Solid Edge part; units mm, degrees
sketch "Sketch1" plane through (0, 0, 0) normal (0, 0, 1) x (1, 0, 0)
  circle A0 centre (0, 0) radius 101.5
extrude "Protrusion1" add sketch "Sketch1" against normal blind 19
sketch "Sketch2" plane through (0, 0, 0) normal (0, 0, 1) x (1, 0, 0)
  circle A0 centre (0, 0) radius 32
extrude "ExtrudedProtrusion_2" add sketch "Sketch2" along normal blind 51
sketch "Sketch3" plane through (0, 0, 0) normal (0, 0, 1) x (1, 0, 0)
  circle A0 centre (0, 0) radius 16
extrude "ExtrudedCutout_1" cut sketch "Sketch3" along normal blind 51 and the other way blind 19
sketch "Sketch4" plane through (0, 0, 0) normal (0, 0, 1) x (1, 0, 0)
  circle A0 centre (0, 86) radius 8
extrude "ExtrudedCutout_2" cut sketch "Sketch4" against normal blind 19
pattern_circular "Pattern1" count 6 over 360 about axis through (0, 0, 0) along (0, 0, -1) of "ExtrudedCutout_2"
sketch "Sketch5" plane through (0, 0, 0) normal (-0.866, -0.5, 0) x (0, 0, -1)
  line L0 (-17.8752, -123.9402) -> (-51, -32)
  line L1 (-51, -32) -> (-51, -21.8003)
  line L2 (19, -21.8003) -> (-51, -21.8003)
  line L3 (19, -117.5) -> (19, -21.8003)
  arc A0 (19, -117.5) -> (-17.8752, -123.9402) centre (0, -117.5) cw
extrude "Protrusion_3" add sketch "Sketch5" along normal mid plane 16
sketch "Sketch6" plane through (0, 0, 0) normal (-0.866, -0.5, 0) x (0, 0, -1)
  circle A0 centre (0, -117.5) radius 6.5
extrude "Cutout_3" cut sketch "Sketch6" along normal mid plane 16
pattern_circular "Pattern2" count 3 over 360 about axis through (0, 0, 0) along (0, 0, -1) of "Protrusion_3", "Cutout_3"
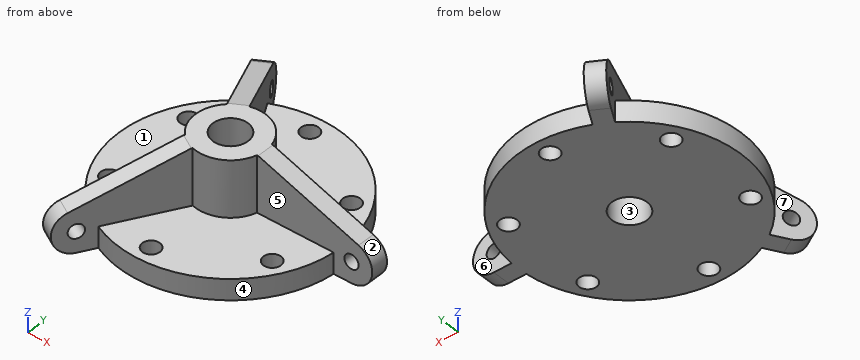
Design review of the part built by this model. Coordinates are the model's own, in mm. Face numbers are marked on the shaded views. A direction names the side the tool comes from. Round coordinates to 2 decimals unless told otherwise and drop trailing zeros. Write each loop counter-clockwise with the first axis right and the second up, starting at its lowest first coordinate (ties: lowest second). Pieces come first, ordered by that corner, then holes. Notation, with made-up numbers: M -30.75,-34 L -8.75,-34 A13 ccw -8.75,-30 Z; hole C -4,-28 d5. An arc over 180 degrees is marked long. One line per item, written item: value. Start each with the question number.
1. Take a section at A-A on y = 0. State the section outline as (x, z) points.
2. Take a section at C-C on z = 13. State the section outline as (x, y) points, then the cut area to 3 significant figures.
3. To check wall thickness, follow probe 1 along Y at (x, z) = (0, -14); probe 2 along X at (y, z) = (-46.5, -4); probe 3 along Z at (x, y) = (92.5, 38.5). State the ranges of each line that lie inside material, in increasing order. Write a range as from..to.
4. Draft analysis for pull direction X (two halves, no side actions). For the marked faces 1, 2, 3 and 4, state which applies: pulls with the +X half, pulls with the -X half, needs draft (parallel to the pull), parting line crosses it, or undercut.
5. Take a section at D-D on y = 43. State the section outline as (x, z) points.
6. Clearance check with flat-ended pins moving along their axes: P1, Ø12, axis at x = 54.5, z = 17, coming from the -Y side; P2, Ø9.5, axis at x = 0, y = -86, coming from the +Z side; P3, Ø8, axis at x = 47.5, z = -9, coming from the +Y side; P4, Ø21, axis at x = 74.48, y = -43, coming from the -Z side. State where each tip first meets the part, or that it passes through.
7. Take a section at B-B on x = 0. State the section outline as (y, z) points, then the cut area to 3 significant figures.
8. For the marked faces 5, 6 and 7, list the 3-axis set-ups (+Z, -Z, +X, -X, +Y, -Y) from which the entire face can be reached by the end or side of a thin tool; tool diameter is ignored.
Computed:
1. outline: M -101.5,-19 L -16,-19 L -16,51 L -32,51 L -32,0 L -101.5,0 Z; M 16,-19 L 117.5,-19 A19 ccw 123.94,17.88 L 32,51 L 16,51 Z; hole C 117.5,0 d13
2. outline: M -72.61,-109.76 L -58.75,-117.76 L -8.56,-30.83 A32 ccw 30.98,-8 L 131.36,-8 L 131.36,8 L 30.98,8 A32 ccw -8.56,30.83 L -58.75,117.76 L -72.61,109.76 L -22.42,22.83 A32 ccw -22.42,-22.83 Z; hole C 0,0 d32
2. area: 7,200 mm²
3. probe 1: y = -101.5..-94, -78..-16, 16..78, 94..101.5
3. probe 2: x = -90.22..-81.67, -67.28..67.28, 81.67..90.22
3. probe 3: z = -19..0
4. face 1: needs draft
4. face 2: pulls with the +X half
4. face 3: undercut
4. face 4: undercut
5. outline: M -91.94,-19 L -82.48,-19 L -82.48,0 L -91.94,0 Z; M -66.48,-19 L 66.48,-19 L 66.48,0 L -15.59,0 L -15.59,46.3 L -34.06,42.98 L -34.06,0 L -66.48,0 Z; M 82.48,-19 L 91.94,-19 L 91.94,0 L 82.48,0 Z
6. P1: stops at y = -8
6. P2: passes through
6. P3: stops at y = 91.71
6. P4: stops at z = -19
7. outline: M -101.5,-19 L -94,-19 L -94,0 L -101.5,0 Z; M -78,-19 L -16,-19 L -16,51 L -32,51 L -32,0 L -78,0 Z; M 16,-19 L 78,-19 L 78,0 L 32,0 L 32,51 L 16,51 Z; M 94,-19 L 101.5,-19 L 101.5,0 L 94,0 Z
7. area: 4,270 mm²
8. face 5: +Z, +X, -Y
8. face 6: +Z, +X, +Y
8. face 7: +Z, -X
